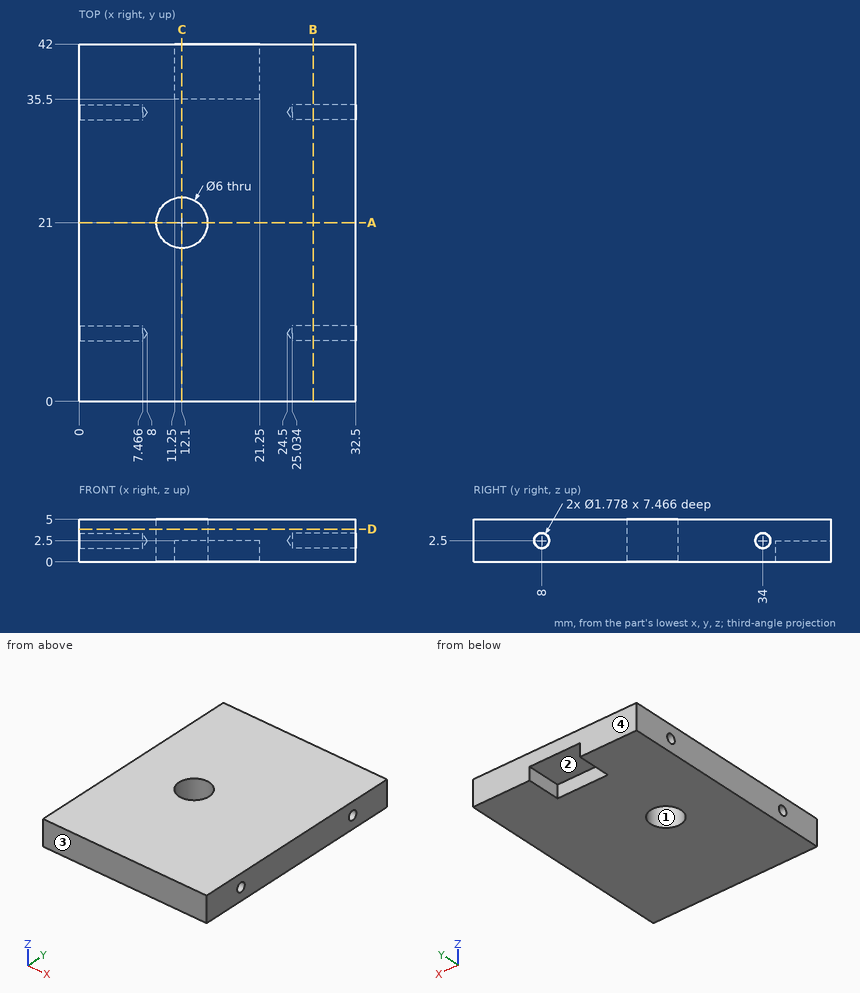
Verification items for this drawing (mm, ordinates from the low corner). Coordinates: 2 decimals unless noted, no trailing zeros. Write each loop counter-clockwise with the first axis right and the second up, starting at its lowest first coordinate (ties: lowest second). Pieces come first, ordered by that corner, then holes. Notation, with made-up numbers: M 10,25 L 49,25 A13 cw 49,50 Z; hole C 6,-38.5 d2. An arc over 180 degrees is marked long. Use one line per item in the form item = value. Start each with the question number.
1) Go/stop test with flat-tipped pins: pin 1 Ø2 at (x, y) = (17.5, 38) entering from -Z; pin 2 Ø1.1 at (y, z) = (8, 2.5) entering from -X; pin 3 Ø1.1 at (y, z) = (8, 2.5) entering from +X. Record where each tip stops, or that it passes through.
2) Section check C-C on x = 12.1. Enter the section's corners in (y, z), and give its area (3 significant figures).
3) Section check B-B on x = 27.5. Enter the section's corners in (y, z), and give its area (3 significant figures).
4) Release check for a two-part mould opening along Y. For the marked faces 1, 2, 3 and 4 record: pulls with the +Y half, pulls with the -Y half, needs draft (parallel to the pull), parting line crosses it, or undercut.
5) Thickness scan on probe 1 along Y at (x, z) = (3.75, 2.5); probe 2 along Z at (x, y) = (2.25, 8); probe 3 along Y at (x, z) = (12.1, 3.95). Record the ranges inside material, lowest first. Write a range as from..to.
6) Section check A-A on y = 21. Enter the section's corners in (x, z).
7) Section check D-D on z = 3.85. Enter the section's corners in (x, y).
Responses:
q1.pin_1 = 2.5
q1.pin_2 = 7.67
q1.pin_3 = 24.83
q2.outline = M 0,0 L 18,0 L 18,5 L 0,5 Z; M 24,0 L 35.5,0 L 35.5,2.5 L 42,2.5 L 42,5 L 24,5 Z
q2.area = 164 mm2
q3.outline = M 0,0 L 42,0 L 42,5 L 0,5 Z; hole C 8,2.5 d1.78; hole C 34,2.5 d1.78
q3.area = 205 mm2
q4.face_1 = undercut
q4.face_2 = needs draft
q4.face_3 = pulls with the -Y half
q4.face_4 = pulls with the +Y half
q5.probe_1 = 0..7.11, 8.89..33.11, 34.89..42
q5.probe_2 = 0..1.61, 3.39..5
q5.probe_3 = 0..18, 24..42
q6.outline = M 0,0 L 9.1,0 L 9.1,5 L 0,5 Z; M 15.1,0 L 32.5,0 L 32.5,5 L 15.1,5 Z
q7.outline = M 0,0 L 32.5,0 L 32.5,42 L 0,42 Z; hole C 12.1,21 d6
